```python
from build123d import *

# Parameters (mm, degrees)
SKETCH_1_R      = 50
SKETCH_1_R_2    = 8.5
SKETCH_1_R_3    = 2.5
EXTRUDE_1_DEPTH = 15


with BuildPart() as part:
    # 草圖1 → 填料-伸長1 (new body)
    with BuildSketch(Plane(origin=(0, 0, 0), x_dir=(0, 0, -1), z_dir=(1, 0, 0))):
        Circle(SKETCH_1_R)
        with Locations((17.320508076, 30)):
            Circle(SKETCH_1_R_2, mode=Mode.SUBTRACT)
        with Locations((34.641016151, 0)):
            Circle(SKETCH_1_R_2, mode=Mode.SUBTRACT)
        with Locations((17.320508076, -30)):
            Circle(SKETCH_1_R_2, mode=Mode.SUBTRACT)
        with Locations((-17.320508076, -30)):
            Circle(SKETCH_1_R_2, mode=Mode.SUBTRACT)
        with Locations((-34.641016151, 0)):
            Circle(SKETCH_1_R_2, mode=Mode.SUBTRACT)
        with Locations((-17.320508076, 30)):
            Circle(SKETCH_1_R_2, mode=Mode.SUBTRACT)
        Circle(SKETCH_1_R_3, mode=Mode.SUBTRACT)
    extrude(amount=EXTRUDE_1_DEPTH)


solid = part.part
```
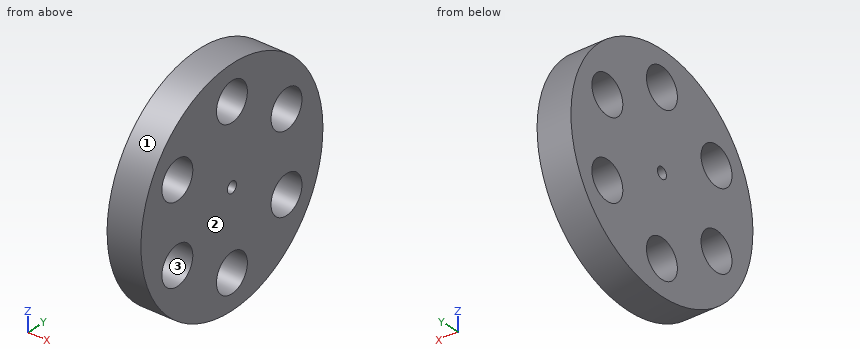
Model file for the job. Use its own axes, mm. Face numbers are marked on the shaded views. Give positions to 0.01 mm unless a question says otherwise; leave off trailing zeros. Write each loop counter-clockwise with the first axis right and the second up, starting at its lowest first coordinate (ties: lowest second). Pieces come first, ordered by that corner, then holes. Notation, with made-up numbers: M 2,39 L 47,39 A27 ccw 47,58 Z; hole C -30,-3.75 d2. An arc over 180 degrees is marked long. Use a Markdown table: item, result.
1) Cut at A-A (z = -14). List the corners of the cut face in (x, y).
Responses:
| item | result |
|---|---|
| outline | M 0,-48 L 15,-48 L 15,-37.82 L 0,-37.82 Z; M 0,-22.18 L 15,-22.18 L 15,22.18 L 0,22.18 Z; M 0,37.82 L 15,37.82 L 15,48 L 0,48 Z |
2) Cut at D-D (z = 0). List the corners of the cut face in (x, y).
Responses:
| item | result |
|---|---|
| outline | M 0,-50 L 15,-50 L 15,-2.5 L 0,-2.5 Z; M 0,2.5 L 15,2.5 L 15,50 L 0,50 Z |
3) Drill centre lines: line 1 (Z direction, x = 14.5, y = -34); line 2 (Z direction, x = 7.5, y = 7); line 3 (Z direction, x = 3.25, y = 1.5). Where is each one in solid material? Low to high. Write a range as from..to.
Responses:
| item | result |
|---|---|
| line 1 | z = -36.66..-24.82, -9.82..9.82, 24.82..36.66 |
| line 2 | z = -49.51..-39.46, -29.82..29.82, 39.46..49.51 |
| line 3 | z = -49.98..-43.01, -26.27..-2, 2..26.27, 43.01..49.98 |
4) Cut at C-C (y = 5). List the corners of the cut face in (x, z), and give its area (3 significant figures).
Responses:
| item | result |
|---|---|
| outline | M 0,-49.75 L 15,-49.75 L 15,-41.51 L 0,-41.51 Z; M 0,-27.77 L 15,-27.77 L 15,27.77 L 0,27.77 Z; M 0,41.51 L 15,41.51 L 15,49.75 L 0,49.75 Z |
| area | 1,080 mm2 |
5) Pull direction Z, two halves, no side cores. Call the marked faces 1, 2 and 3: +Z half, -Z half, draft (parallel to the pull), parting line (faces both ways), or undercut.
Responses:
| item | result |
|---|---|
| face 1 | parting line |
| face 2 | draft |
| face 3 | undercut |
6) Pin check, flat tips, straight feed: pin 1 (15.5 mm diameter, centred on y = 0, z = 34.64, fed in from +X) (3 decimals); pin 2 (4 mm diameter, centred on x = 7, y = -12.5, fed in from -Z); pin 3 (1.5 mm diameter, centred on x = 8.5, y = -21, fed in from +Z); pin 4 (2 mm diameter, centred on x = 11, y = 20, fed in from +Z). Stop position of each tip, or through.
Responses:
| item | result |
|---|---|
| pin 1 | passes through |
| pin 2 | stops at z = -48.89 |
| pin 3 | stops at z = 45.72 |
| pin 4 | stops at z = 46.25 |
7) Cut at B-B (x = 1.5). List the corners of the cut face in (y, z), and give its area (3 significant figures).
Responses:
| item | result |
|---|---|
| outline | C 0,0 d100; hole C -30,-17.32 d17; hole C -30,17.32 d17; hole C 0,-34.64 d17; hole C 0,34.64 d17; hole C 0,0 d5; hole C 30,-17.32 d17; hole C 30,17.32 d17 |
| area | 6,470 mm2 |
